```python
from build123d import *

# Parameters (mm, degrees)
F1_DEPTH = 1524


with BuildPart() as f1:
    # F0 (on Right) → F1 (new body)
    with BuildSketch(Plane.YZ):
        with BuildLine():
            Line((-3.830222, 3.213938), (0, 0))
            Line((0, 0), (57.163184, 68.12443))
            ThreePointArc((57.163184, 68.12443), (102.045095, 235.626002), (2.580983, 377.675475))
            Line((2.580983, 377.675475), (-58.040795, 412.675475))
            ThreePointArc((-58.040795, 412.675475), (-62.700053, 418.747538), (-61.701049, 426.335729))
            Line((-61.701049, 426.335729), (-48.038476, 450))
            Line((-48.038476, 450), (-52.368603, 452.5))
            Line((-52.368603, 452.5), (-66.031176, 428.835729))
            ThreePointArc((-66.031176, 428.835729), (-67.507418, 417.371282), (-60.392876, 408.261062))
            Line((-60.392876, 408.261062), (0.081466, 373.346184))
            ThreePointArc((0.081466, 373.346184), (97.122196, 234.756858), (53.332304, 71.336081))
            Line((53.332304, 71.336081), (-3.830222, 3.213938))
        make_face()
    extrude(amount=F1_DEPTH)


solid = f1.part
```
Work out the finished part from the listing and answer in its coordinate system (mm). Coordinates: 2 decimals unless noted, no trailing zeros. Loops run counter-clockwise (first coordinate to the right, second up) from the corner with the lowest first, then second, coordinate; pieces in that order, holes last. Notation, with made-up numbers: M 55,-17 L 94,-17 A30 cw 94,17 Z; hole C -2.75,-18 d10. An arc over 180 degrees is marked long. Use CSV: the item, a comma, the result in double quotes. Start each with the question number.
(1) Find section A-A, the plane x = 736. Give the vertices of the cut face in (y, z).
(2) Find section C-C, the plane z = 55. Give the vertices of the cut face in (x, y).
(3) Find section B-B, the plane y = 22. Give the vertices of the cut face in (x, z).
(4) For a pull along Z with two mould halves and no side action, classify faces 1 (the face through (751.332, 102.465, 233.155)), 2 (the face through (751.33, 25.15, 37.75)), 3 (the face through (0, 102, 227)) as +Z half, -Z half, draft (parallel to the pull), parting line (faces both ways), or undercut.
(5) Given pin 1 Ø1.5 at (x, z) = (1292, 341) entering from -Y; pin 2 Ø1 at (x, y) = (960, -30) entering from +Z; pin 3 Ø2 at (x, z) = (1035, 347) entering from +Y, each flat-ended and moving along its own axis, determine where each tip first touches the part or whether it passes through.
(6) Find section D-D, the plane y = -34. Give the vertices of the cut face in (x, z), then the cut area to 3 significant figures.
(7) Consider line 1 (Z direction, x = 1163, y = -2.5); line 2 (Z direction, x = 672, y = 52); line 3 (Y direction, x = 858.5, z = 407). Determine where each line is inside the solid, lowest interval first.
Recorded:
1,outline,"M -66.03,428.84 A15 ccw -60.39,408.26 L 0.08,373.35 A200.16 cw 53.33,71.34 L -3.83,3.21 L 0,0 L 57.16,68.12 A205.16 ccw 2.58,377.68 L -58.04,412.68 A10 cw -61.7,426.34 L -48.04,450 L -52.37,452.5 Z"
2,outline,"M 0,39.62 L 1524,39.62 L 1524,46.15 L 0,46.15 Z"
3,outline,"M 0,26.22 L 1524,26.22 L 1524,34 L 0,34 Z; M 0,358.69 L 1524,358.69 L 1524,364.95 L 0,364.95 Z"
4,face 1,"parting line"
4,face 2,"undercut"
4,face 3,"draft"
5,pin 1,"stops at y = 41.32"
5,pin 2,"stops at z = 396.77"
5,pin 3,"stops at y = 44.14"
6,outline,"M 0,393.02 L 1524,393.02 L 1524,398.8 L 0,398.8 Z"
6,area,"8,800 mm^2"
7,line 1,"z = 2.1 to 4.8, 374.84 to 380.61"
7,line 2,"z = 61.97 to 69.75, 330.24 to 337.79"
7,line 3,"y = -58.21 to -48.21"
